```python
from build123d import *

# Parameters (mm, degrees)
EXTRUDE_THIN2_DEPTH = 139.7
CUT_EXTRUDE1_DEPTH  = 150.568174674


with BuildPart() as part:
    # Sketch1 → Extrude-Thin2 (new body)
    with BuildSketch(Plane(origin=(0, 0, 0), x_dir=(0, 0, -1), z_dir=(1, 0, 0))):
        with BuildLine():
            Line((-39.935482404, 37.455825651), (-71.685482404, 37.455825651))
            ThreePointArc((-71.685482404, 37.455825651), (-73.930546435, 36.525889681), (-74.860482404, 34.280825651))
            Line((-74.860482404, 34.280825651), (-74.860482404, -10.169174349))
            ThreePointArc((-74.860482404, -10.169174349), (-73.930546435, -12.414238379), (-71.685482404, -13.344174349))
            Line((-71.685482404, -13.344174349), (-39.935482404, -13.344174349))
            ThreePointArc((-39.935482404, -13.344174349), (-37.690418374, -12.414238379), (-36.760482404, -10.169174349))
            Line((-36.760482404, -10.169174349), (-36.760482404, 34.280825651))
            ThreePointArc((-36.760482404, 34.280825651), (-37.690418374, 36.525889681), (-39.935482404, 37.455825651))
        make_face()
        with BuildLine():
            Line((-39.935482404, 35.804825651), (-71.685482404, 35.804825651))
            ThreePointArc((-71.685482404, 35.804825651), (-72.763113139, 35.358456386), (-73.209482404, 34.280825651))
            Line((-73.209482404, 34.280825651), (-73.209482404, -10.169174349))
            ThreePointArc((-73.209482404, -10.169174349), (-72.763113139, -11.246805083), (-71.685482404, -11.693174349))
            Line((-71.685482404, -11.693174349), (-39.935482404, -11.693174349))
            ThreePointArc((-39.935482404, -11.693174349), (-38.85785167, -11.246805083), (-38.411482404, -10.169174349))
            Line((-38.411482404, -10.169174349), (-38.411482404, 34.280825651))
            ThreePointArc((-38.411482404, 34.280825651), (-38.85785167, 35.358456386), (-39.935482404, 35.804825651))
        make_face(mode=Mode.SUBTRACT)
    extrude(amount=EXTRUDE_THIN2_DEPTH)

    # Sketch3 → Cut-Extrude1 (cut, through all)
    with BuildSketch(Plane.XY.offset(74.860482404)):
        Polygon((0, 37.455825651), (0, -38.744174349), (76.2, -38.744174349), align=None)
        Polygon((139.7, 37.455825651), (81.28, -20.964174349), (139.7, -20.964174349), align=None)
    extrude(amount=-CUT_EXTRUDE1_DEPTH, mode=Mode.SUBTRACT)


solid = part.part
```
Input: part model. Units: mm. Frame: model coordinates. A direction names the side the tool comes from. Coordinates: 2 decimals unless noted, no trailing zeros. Loops run counter-clockwise (first coordinate to the right, second up) from the corner with the lowest first, then second, coordinate; pieces in that order, holes last. Notation, with made-up numbers: (-39, 8) - (-15, 8) arc R29 cw to (-15, 35) - close; hole circle Ø4 at (83, -13.5). An arc over 180 degrees is marked (long way). Answer in a Markdown table with one row per item.
(1) Mould query, pull axis Z, two halves, no side actions, for faces 3 (the face through (114.419, 12.174, 74.244)), 4 (the face through (69.539, -12.439, 37.715)), 5 (the face through (69, 17, 73.209)). Classes: pulls with the +Z half, pulls with the -Z half, needs draft (parallel to the pull), parting line crosses it, or undercut.
Model answer:
| item | result |
|---|---|
| face 3 | needs draft |
| face 4 | pulls with the -Z half |
| face 5 | undercut |
(2) Cut plane B-B on y = 20. Output: boundary loops of the cut face in (x, z), plus the area to 3 significant figures.
Model answer:
| item | result |
|---|---|
| outline | (17.46, 36.76) - (122.24, 36.76) - (122.24, 38.41) - (17.46, 38.41) - close; (17.46, 73.21) - (122.24, 73.21) - (122.24, 74.86) - (17.46, 74.86) - close |
| area | 346 mm² |
(3) Cut plane D-D on x = 15. Output: boundary loops of the cut face in (y, z) (3 decimals), plus the area to 3 significant figures.
Model answer:
| item | result |
|---|---|
| outline | (22.456, 36.76) - (34.281, 36.76) arc R3.175 ccw to (37.456, 39.935) - (37.456, 71.685) arc R3.175 ccw to (34.281, 74.86) - (22.456, 74.86) - (22.456, 73.209) - (34.281, 73.209) arc R1.524 cw to (35.805, 71.685) - (35.805, 39.935) arc R1.524 cw to (34.281, 38.411) - (22.456, 38.411) - close |
| area | 104 mm² |
(4) Cut plane C-C on x = 62.5. Output: boundary loops of the cut face in (y, z) (3 decimals).
Model answer:
| item | result |
|---|---|
| outline | (-13.344, 39.935) arc R3.175 ccw to (-10.169, 36.76) - (34.281, 36.76) arc R3.175 ccw to (37.456, 39.935) - (37.456, 71.685) arc R3.175 ccw to (34.281, 74.86) - (-10.169, 74.86) arc R3.175 ccw to (-13.344, 71.685) - close; hole (-11.693, 39.935) arc R1.524 ccw to (-10.169, 38.411) - (34.281, 38.411) arc R1.524 ccw to (35.805, 39.935) - (35.805, 71.685) arc R1.524 ccw to (34.281, 73.209) - (-10.169, 73.209) arc R1.524 ccw to (-11.693, 71.685) - close |
(5) Set-up query: faces 1 (the face through (69, 37.456, 56)), 2 (the face through (69, 35.805, 56)). Return all of +Z, -Z, +X, -X, +Y, -Y with unobstructed straight access to the full face (end or side cutting, diameter ignored); none if empty.
Model answer:
| item | result |
|---|---|
| face 1 | +Z, -Z, +X, -X, +Y |
| face 2 | +X, -X |
(6) Pin query (flat end, axial travel): P1, Ø6, axis at x = 35, z = 61.5, coming from the -Y side. Return the tip coordinate at first contact, or that it passes through.
Model answer:
| item | result |
|---|---|
| P1 | stops at y = 35.8 |
(7) Material intervals for L1, parallel to Z at x = 126.5, y = 30; L2, parallel to Y at x = 51, z = 67.5; L3, parallel to Y at x = 111.5, z = 51, sorted ascending. Write a range as from..to.
Model answer:
| item | result |
|---|---|
| L1 | z = 36.76..38.41, 73.21..74.86 |
| L2 | y = -13.34..-11.69, 35.8..37.46 |
| L3 | y = 35.8..37.46 |
(8) Cut plane A-A on z = 68.5. Output: boundary loops of the cut face in (x, y), plus the area to 3 significant figures.
Model answer:
| item | result |
|---|---|
| outline | (0, 37.46) - (1.65, 35.8) - (138.05, 35.8) - (139.7, 37.46) - close; (49.15, -11.69) - (50.8, -13.34) - (88.9, -13.34) - (90.55, -11.69) - close |
| area | 294 mm² |
